Part model, mm, in its own coordinate system. Face numbers are marked on the shaded views. A direction names the side the tool comes from. Coordinates: 2 decimals unless noted, no trailing zeros. Loops run counter-clockwise (first coordinate to the right, second up) from the corner with the lowest first, then second, coordinate; pieces in that order, holes last. Notation, with made-up numbers: (-27.75, 59) - (-9.75, 59) arc R24 cw to (-9.75, 70) - close; hole circle Ø5 at (87, 15.25). An arc over 180 degrees is marked (long way). Use a Markdown table: item, result. Add a question column.
1. Band-saw the part on C-C, the plane x = 40.5. Give the cut face in (y, z), plus the area to 3 significant figures.
2. Wall check: probe 1 along X at (y, z) = (-0.75, -8.25); probe 2 along X at (y, z) = (10, -3); probe 3 along Y at (x, z) = (-14, -0.75). Give the ranges that are in metal, low to high. Write a range as [from, to].
3. Band-saw the part on A-A, the plane y = 0. Give the cut face in (x, z), plus the area to 4 significant figures.
4. Drop flat-ended pins along their axis: pin 1 (10 mm diameter, centred on x = -16, y = 11, fed in from -Z); pin 2 (2 mm diameter, centred on x = 19, z = 3, fed in from -Y); pin 3 (3 mm diameter, centred on x = 1, z = -7.5, fed in from -Y). Give the stop position or say it passes through.
5. Band-saw the part on D-D, the plane x = 29. Give the cut face in (y, z).
6. 3-axis set-ups, long thin cutter, end or side, ignore diameter. For the marked faces 1 and 2: which of +Z, -Z, +X, -X, +Y, -Y reach the whole face in a straight line?
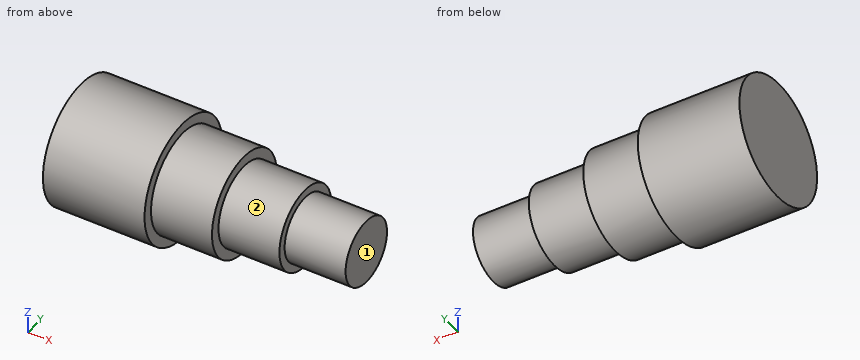
from build123d import *

# Parameters (mm, degrees)
F0_R     = 15
F1_DEPTH = 25
F2_R     = 12.5
F3_DEPTH = 15
F4_R     = 10
F5_DEPTH = 15
F6_R     = 8
F7_DEPTH = 15


# Not quite as in the source:
# - the program builds the solid bodies; features that only make, move or delete a surface that nothing else refers to are left out


with BuildPart() as f1:
    # F0 (on Right) → F1 (new body)
    with BuildSketch(Plane.YZ):
        Circle(F0_R)
    extrude(amount=-F1_DEPTH)

    # F2 (on face) → F3 (join)
    with BuildSketch(Plane.YZ):
        Circle(F2_R)
    extrude(amount=F3_DEPTH)

    # F4 (on face) → F5 (join)
    with BuildSketch(Plane.YZ.offset(15)):
        Circle(F4_R)
    extrude(amount=F5_DEPTH)

    # F6 (on face) → F7 (join)
    with BuildSketch(Plane.YZ.offset(30)):
        Circle(F6_R)
    extrude(amount=F7_DEPTH)


solid = f1.part
Geometry check:
| question | item | result |
|---|---|---|
| 1 | outline | circle Ø16 at (0, 0) |
| 1 | area | 201 mm^2 |
| 2 | probe 1 | x = [-25, 30] |
| 2 | probe 2 | x = [-25, 15] |
| 2 | probe 3 | y = [-14.98, 14.98] |
| 3 | outline | (-25, -15) - (0, -15) - (0, -12.5) - (15, -12.5) - (15, -10) - (30, -10) - (30, -8) - (45, -8) - (45, 8) - (30, 8) - (30, 10) - (15, 10) - (15, 12.5) - (0, 12.5) - (0, 15) - (-25, 15) - close |
| 3 | area | 1,665 mm^2 |
| 4 | pin 1 | stops at z = -13.75 |
| 4 | pin 2 | stops at y = -9.8 |
| 4 | pin 3 | stops at y = -13.57 |
| 5 | outline | circle Ø20 at (0, 0) |
| 6 | face 1 | +Z, -Z, +X, +Y, -Y |
| 6 | face 2 | +X |
